Answer from the drawing. Dimensions are ordinates in mm from the lowest x, y and z of the part. Round coordinates to 2 decimals unless told otherwise and drop trailing zeros. Loops run counter-clockwise (first coordinate to the right, second up) from the corner with the lowest first, then second, coordinate; pieces in that order, holes last.
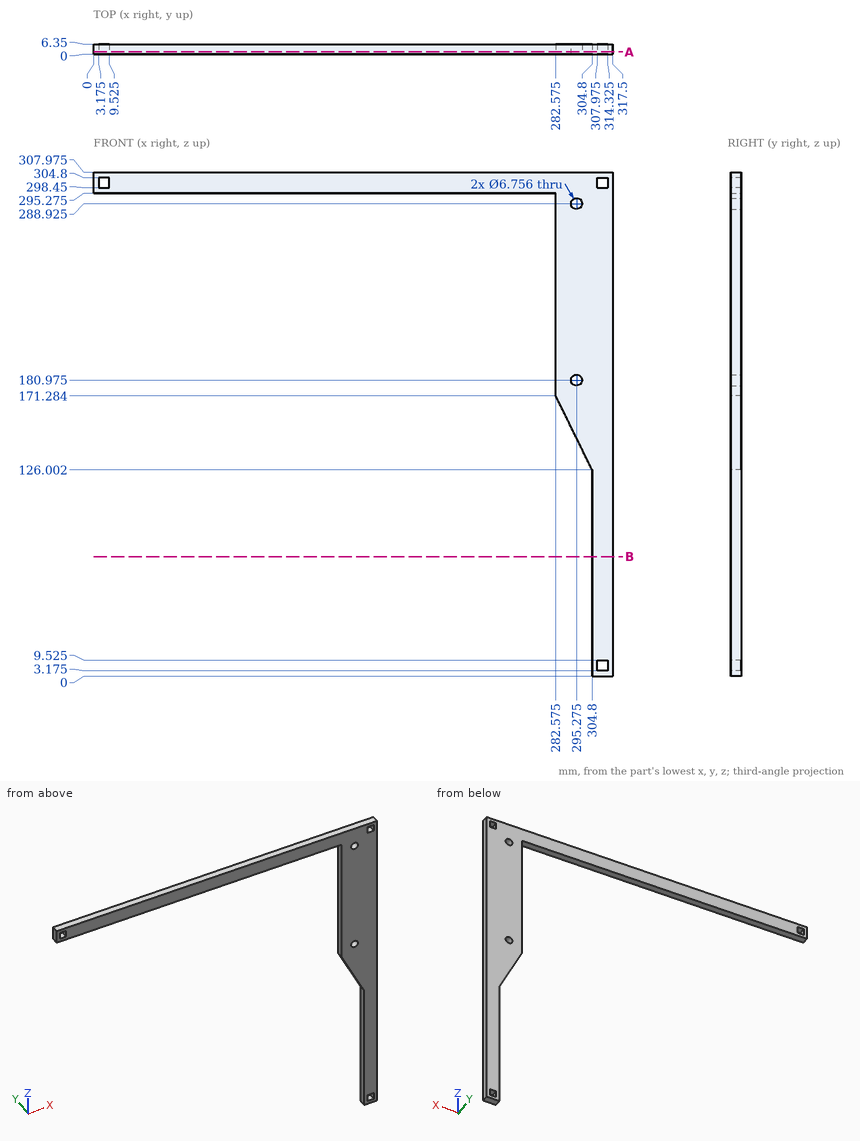
Item 1: Section A-A, the plane y = 1.5 is taken. State how many separate pieces and enclosed holes the cut face has, plus the area to 3 significant figures.
Item 2: Each of these flat-tipped pins is pushed along its axis until it touches: P1, Ø3, axis at x = 126, y = 2, coming from the -Z side (3 decimals); P2, Ø1.9, axis at y = 3, z = 70, coming from the -X side. Where does it stop, or does it pass through?
Item 3: Section B-B, the plane z = 73 is taken. Give the vertices of the cut face in (x, y).
Item 4: Straight lines are drawn through the part: line 1 (Z direction, x = 278, y = 4.5) (1 decimal); line 2 (X direction, y = 3.5, z = 91.5); line 3 (X direction, y = 6, z = 274.5) (1 decimal). For each, find the intervals that lie inside material, in ascending order.
Answer below:
1. separate pieces: 1
1. enclosed holes: 5
1. area: 10,800 mm2
2. P1: stops at z = 295.275
2. P2: stops at x = 304.8
3. outline: (304.8, 0) - (317.5, 0) - (317.5, 6.35) - (304.8, 6.35) - close
4. line 1: z = 295.3 to 308
4. line 2: x = 304.8 to 317.5
4. line 3: x = 282.6 to 317.5
